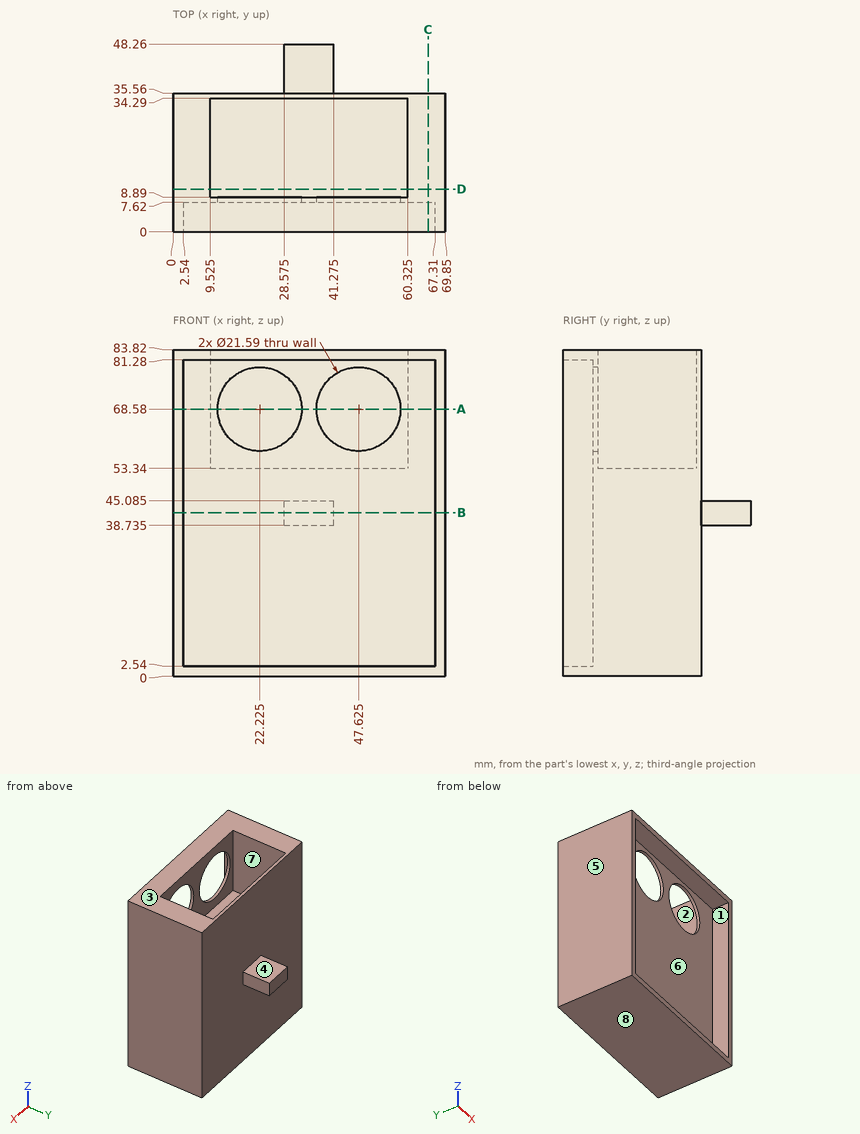
Design review of the part shown in the three views and the two pictorial views. Dimensions are in mm from the part's minimum x, y and z. A direction names the side the tool comes from. Give positions to 0.01 mm unless a question says otherwise; leave off trailing zeros. Loops run counter-clockwise (first coordinate to the right, second up) from the corner with the lowest first, then second, coordinate; pieces in that order, holes last. Notation, with made-up numbers: (-7, -30) -> (38, -30) arc R28 cw to (38, 2) -> close; hole circle Ø6 at (45, 71.5). An arc over 180 degrees is marked (long way). Write each question's results on one line, items separated by ' | '.
Q1. Take a section at D-D, the plane y = 11. Write out the cut boundary in (x, z) (3 decimals).
Reply:
outline: (0, 0) -> (69.85, 0) -> (69.85, 83.82) -> (60.325, 83.82) -> (60.325, 53.34) -> (9.525, 53.34) -> (9.525, 83.82) -> (0, 83.82) -> close
Q2. Wall thickness on L1, parallel to X at y = 8, z = 68; L2, parallel to Z at x = 61.5, y = 5; L3, parallel to X at y = 6, z = 58.5: over which ranges is each line inside the solid? List them lowest first.
Reply:
L1: x = 0 to 11.45, 33 to 36.85, 58.4 to 69.85 | L2: z = 0 to 2.54, 81.28 to 83.82 | L3: x = 0 to 2.54, 67.31 to 69.85
Q3. For pin 1 Ø12 at (x, z) = (54.5, 53.5) entering from +Y; pin 2 Ø2.5 at (x, y) = (40, 4) entering from -Z; pin 3 Ø6 at (x, z) = (57.5, 38.5) entering from -Y; pin 4 Ø12.5 at (x, y) = (38.5, 22.5) entering from +Z, all flat-tipped, find the tip position at first contact; note any pin that passes through.
Reply:
pin 1: stops at y = 35.56 | pin 2: stops at z = 0 | pin 3: stops at y = 7.62 | pin 4: stops at z = 53.34
Q4. Machinability: for the marked faces 4, 5, 6, 7 and 8, which of the approach directions +Z, -Z, +X, -X, +Y, -Y give a long, thin tool a straight path to every point of the face, cutting with its end or side? Answer none if there is none.
Reply:
face 4: +Z, +X, -X, +Y | face 5: +Z, -Z, -X, +Y, -Y | face 6: -Y | face 7: +Z | face 8: -Z, +X, -X, +Y, -Y
Q5. Take a section at B-B, the plane z = 42. Write out the cut boundary in (x, y) (3 decimals).
Reply:
outline: (0, 0) -> (2.54, 0) -> (2.54, 7.62) -> (67.31, 7.62) -> (67.31, 0) -> (69.85, 0) -> (69.85, 35.56) -> (41.275, 35.56) -> (41.275, 48.26) -> (28.575, 48.26) -> (28.575, 35.56) -> (0, 35.56) -> close
Q6. Take a section at C-C, the plane x = 65.5. Write out the cut boundary in (y, z), plus the area to 3 significant figures.
Reply:
outline: (0, 0) -> (35.56, 0) -> (35.56, 83.82) -> (0, 83.82) -> (0, 81.28) -> (7.62, 81.28) -> (7.62, 2.54) -> (0, 2.54) -> close | area: 2,380 mm²
Q7. The part is to be moulded in two halves that separate along Z. For the marked faces 1, 2 and 3, say which applies: +Z half, -Z half, draft (parallel to the pull), parting line (faces both ways), or undercut.
Reply:
face 1: undercut | face 2: draft | face 3: +Z half
Q8. Take a section at A-A, the plane z = 68.58. Write out the cut boundary in (x, y) (3 decimals), plus the area to 3 significant figures.
Reply:
outline: (0, 0) -> (2.54, 0) -> (2.54, 7.62) -> (11.43, 7.62) -> (11.43, 8.89) -> (9.525, 8.89) -> (9.525, 34.29) -> (60.325, 34.29) -> (60.325, 8.89) -> (58.42, 8.89) -> (58.42, 7.62) -> (67.31, 7.62) -> (67.31, 0) -> (69.85, 0) -> (69.85, 35.56) -> (0, 35.56) -> close; (33.02, 7.62) -> (36.83, 7.62) -> (36.83, 8.89) -> (33.02, 8.89) -> close | area: 645 mm²
